from build123d import *

# Parameters (mm, degrees)
F0_R     = 88.9
F0_R_2   = 1.5875
F0_R_3   = 15.875
F1_DEPTH = 3.175


with BuildPart() as f1:
    # F0 (on Front) → F1 (new body)
    with BuildSketch(Plane.XZ):
        Circle(F0_R)
        with BuildLine():
            ThreePointArc((13.438712, -30.112803), (6.635493, -54.919861), (-9.469491, -74.977364))
            ThreePointArc((-9.469491, -74.977364), (-13.93913, -74.54891), (-13.510676, -70.079271))
            ThreePointArc((-13.510676, -70.079271), (0.98008, -52.032162), (7.101402, -29.711554))
            ThreePointArc((7.101402, -29.711554), (10.470681, -26.743524), (13.438712, -30.112803))
        make_face(mode=Mode.SUBTRACT)
        with BuildLine():
            ThreePointArc((-19.359097, -26.694667), (-44.244249, -33.206436), (-69.667048, -29.287863))
            ThreePointArc((-69.667048, -29.287863), (-71.530815, -25.202814), (-67.445767, -23.339047))
            ThreePointArc((-67.445767, -23.339047), (-44.571135, -26.864855), (-22.18026, -21.005771))
            ThreePointArc((-22.18026, -21.005771), (-17.92523, -22.439638), (-19.359097, -26.694667))
        make_face(mode=Mode.SUBTRACT)
        with BuildLine():
            ThreePointArc((-3.418136, -32.797809), (-21.713426, -50.879741), (-45.689502, -60.197557))
            ThreePointArc((-45.689502, -60.197557), (-49.346096, -57.591685), (-46.740224, -53.935091))
            ThreePointArc((-46.740224, -53.935091), (-25.167307, -45.551214), (-8.705783, -29.281662))
            ThreePointArc((-8.705783, -29.281662), (-4.303886, -28.395912), (-3.418136, -32.797809))
        make_face(mode=Mode.SUBTRACT)
        with BuildLine():
            ThreePointArc((26.694667, -19.359097), (33.206436, -44.244249), (29.287863, -69.667048))
            ThreePointArc((29.287863, -69.667048), (25.202814, -71.530815), (23.339047, -67.445767))
            ThreePointArc((23.339047, -67.445767), (26.864855, -44.571135), (21.005771, -22.18026))
            ThreePointArc((21.005771, -22.18026), (22.439638, -17.92523), (26.694667, -19.359097))
        make_face(mode=Mode.SUBTRACT)
        with BuildLine():
            ThreePointArc((32.797809, -3.418136), (50.879741, -21.713426), (60.197557, -45.689502))
            ThreePointArc((60.197557, -45.689502), (57.591685, -49.346096), (53.935091, -46.740224))
            ThreePointArc((53.935091, -46.740224), (45.551214, -25.167307), (29.281662, -8.705783))
            ThreePointArc((29.281662, -8.705783), (28.395912, -4.303886), (32.797809, -3.418136))
        make_face(mode=Mode.SUBTRACT)
        with Locations((0, -22.225)):
            Circle(F0_R_2, mode=Mode.SUBTRACT)
        with BuildLine():
            ThreePointArc((30.112803, 13.438712), (54.919861, 6.635493), (74.977364, -9.469491))
            ThreePointArc((74.977364, -9.469491), (74.54891, -13.93913), (70.079271, -13.510676))
            ThreePointArc((70.079271, -13.510676), (52.032162, 0.98008), (29.711554, 7.101402))
            ThreePointArc((29.711554, 7.101402), (26.743524, 10.470681), (30.112803, 13.438712))
        make_face(mode=Mode.SUBTRACT)
        with BuildLine():
            ThreePointArc((-30.112803, -13.438712), (-54.919861, -6.635493), (-74.977364, 9.469491))
            ThreePointArc((-74.977364, 9.469491), (-74.54891, 13.93913), (-70.079271, 13.510676))
            ThreePointArc((-70.079271, 13.510676), (-52.032162, -0.98008), (-29.711554, -7.101402))
            ThreePointArc((-29.711554, -7.101402), (-26.743524, -10.470681), (-30.112803, -13.438712))
        make_face(mode=Mode.SUBTRACT)
        with Locations((-22.225, 0)):
            Circle(F0_R_2, mode=Mode.SUBTRACT)
        with BuildLine():
            ThreePointArc((-32.797809, 3.418136), (-50.879741, 21.713426), (-60.197557, 45.689502))
            ThreePointArc((-60.197557, 45.689502), (-57.591685, 49.346096), (-53.935091, 46.740224))
            ThreePointArc((-53.935091, 46.740224), (-45.551214, 25.167307), (-29.281662, 8.705783))
            ThreePointArc((-29.281662, 8.705783), (-28.395912, 4.303886), (-32.797809, 3.418136))
        make_face(mode=Mode.SUBTRACT)
        with BuildLine():
            ThreePointArc((-26.694667, 19.359097), (-33.206436, 44.244249), (-29.287863, 69.667048))
            ThreePointArc((-29.287863, 69.667048), (-25.202814, 71.530815), (-23.339047, 67.445767))
            ThreePointArc((-23.339047, 67.445767), (-26.864855, 44.571135), (-21.005771, 22.18026))
            ThreePointArc((-21.005771, 22.18026), (-22.439638, 17.92523), (-26.694667, 19.359097))
        make_face(mode=Mode.SUBTRACT)
        Circle(F0_R_3, mode=Mode.SUBTRACT)
        with Locations((22.225, 0)):
            Circle(F0_R_2, mode=Mode.SUBTRACT)
        with Locations((0, 22.225)):
            Circle(F0_R_2, mode=Mode.SUBTRACT)
        with BuildLine():
            ThreePointArc((3.418136, 32.797809), (21.713426, 50.879741), (45.689502, 60.197557))
            ThreePointArc((45.689502, 60.197557), (49.346096, 57.591685), (46.740224, 53.935091))
            ThreePointArc((46.740224, 53.935091), (25.167307, 45.551214), (8.705783, 29.281662))
            ThreePointArc((8.705783, 29.281662), (4.303886, 28.395912), (3.418136, 32.797809))
        make_face(mode=Mode.SUBTRACT)
        with BuildLine():
            ThreePointArc((19.359097, 26.694667), (44.244249, 33.206436), (69.667048, 29.287863))
            ThreePointArc((69.667048, 29.287863), (71.530815, 25.202814), (67.445767, 23.339047))
            ThreePointArc((67.445767, 23.339047), (44.571135, 26.864855), (22.18026, 21.005771))
            ThreePointArc((22.18026, 21.005771), (17.92523, 22.439638), (19.359097, 26.694667))
        make_face(mode=Mode.SUBTRACT)
        with BuildLine():
            ThreePointArc((-13.438712, 30.112803), (-6.635493, 54.919861), (9.469491, 74.977364))
            ThreePointArc((9.469491, 74.977364), (13.93913, 74.54891), (13.510676, 70.079271))
            ThreePointArc((13.510676, 70.079271), (-0.98008, 52.032162), (-7.101402, 29.711554))
            ThreePointArc((-7.101402, 29.711554), (-10.470681, 26.743524), (-13.438712, 30.112803))
        make_face(mode=Mode.SUBTRACT)
    extrude(amount=-F1_DEPTH)


solid = f1.part
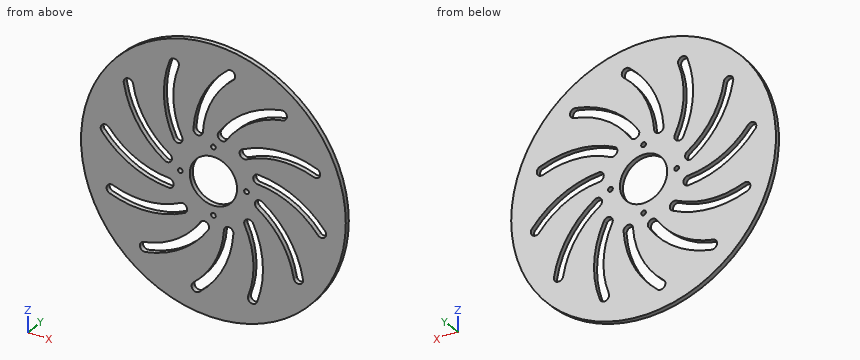
The listing builds one solid part. Answer for the finished solid, in the listing's coordinates (mm). Give positions to 0.01 mm unless a question says otherwise; leave off trailing zeros. Loops run counter-clockwise (first coordinate to the right, second up) from the corner with the lowest first, then second, coordinate; pieces in that order, holes last. Notation, with made-up numbers: (62, -23) - (117, -23) arc R8 ccw to (117, -12) - close; hole circle Ø6 at (31.25, 47). An arc over 180 degrees is marked (long way). Write each question's results on one line, items separated by ' | '.
1. Flat-ended cylindrical pins translate along their axes: P1, Ø5, axis at x = -48, z = 34, coming from the -Y side; P2, Ø3, axis at x = 0, z = 22.225, coming from the -Y side. Find the tip coordinate at first contact, or state that the pin passes through.
Resolved:
P1: stops at y = 0 | P2: passes through
2. Consider probe 1 along X at (y, z) = (1.15, 70.5); probe 2 along Z at (x, y) = (0, 2.15) (1 decimal); probe 3 along X at (y, z) = (1.05, -21). Determine where each line is inside the solid, lowest interval first. Write a range as from..to.
Resolved:
probe 1: x = -54.16..-28.82, -23.8..4.59, 13.93..54.16 | probe 2: z = -88.9..-65.3, -53.9..-23.8, -20.6..-15.9, 15.9..20.6, 23.8..53.9, 65.3..88.9 | probe 3: x = -86.38..-22.17, -19.37..-1.01, 1.01..20.68, 27.48..42.58, 50.41..86.38
3. Find section A-A, the plane x = -40.5. Write down the section's boundary in (y, z) (3 decimals), then the cut area to 3 significant figures.
Resolved:
outline: (0, -79.139) - (3.175, -79.139) - (3.175, -59.102) - (0, -59.102) - close; (0, -52.524) - (3.175, -52.524) - (3.175, -32.902) - (0, -32.902) - close; (0, -26.508) - (3.175, -26.508) - (3.175, -11.909) - (0, -11.909) - close; (0, -5.369) - (3.175, -5.369) - (3.175, 9.447) - (0, 9.447) - close; (0, 18.502) - (3.175, 18.502) - (3.175, 79.139) - (0, 79.139) - close | area: 412 mm^2
4. Find section B-B, the plane y = 0.5. Count the separate pieces of the cut face and the enclosed holes in it, then the cut area to 3 significant figures.
Resolved:
separate pieces: 1 | enclosed holes: 17 | area: 19,900 mm^2
